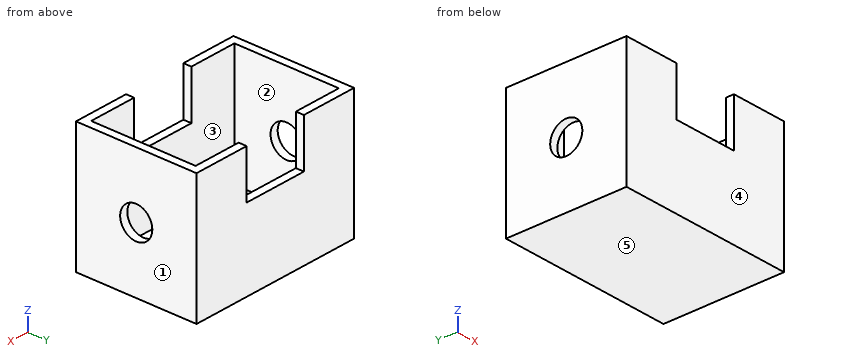
```python
from build123d import *

# Parameters (mm, degrees)
F0_W     = 139.7
F0_H     = 95.25
F1_DEPTH = 101.6
F2_T     = -6.35
F3_W     = 50.8
F3_H     = 38.1
F4_DEPTH = 101.6
F5_R     = 12.7
F6_DEPTH = 177.8


with BuildPart() as f1:
    # F0 (on Top) → F1 (new body)
    with BuildSketch(Plane.XY):
        Rectangle(F0_W, F0_H)
    extrude(amount=F1_DEPTH)

    # F2
    f2_openings = [f1.faces().sort_by_distance(p)[0] for p in [
        (0, 0, 101.6),
    ]]
    offset(amount=F2_T, openings=f2_openings)

    # F3 (on face) → F4 (cut)
    with BuildSketch(Plane.XZ.offset(47.625)):
        with Locations((0, 82.55)):
            Rectangle(F3_W, F3_H)
    extrude(amount=-F4_DEPTH, mode=Mode.SUBTRACT)

    # F5 (on face) → F6 (cut)
    with BuildSketch(Plane.YZ.offset(69.85)):
        with Locations((0, 50.8)):
            Circle(F5_R)
    extrude(amount=-F6_DEPTH, mode=Mode.SUBTRACT)


solid = f1.part
```
Geometry: final body of the model. Coordinates: model frame, mm. Face numbers are marked on the shaded views. A direction names the side the tool comes from. Coordinates: 2 decimals unless noted, no trailing zeros. Order: outer loops, then holes, each group sorted by start corner. A loop starts at its lowest first (then second) coordinate and runs counter-clockwise, first axis right, second up. Notation, with made-up numbers: (-0.5, 27.5) - (44.5, 27.5) arc R26 cw to (44.5, 41.5) - close; hole circle Ø11 at (73.5, 53). An arc over 180 degrees is marked (long way). Write each question's results on one line, items separated by ' | '.
(1) Line query: line 1 (X direction, y = 35.5, z = 52.5); line 2 (Z direction, x = -66.75, y = 0); line 3 (Y direction, x = -55, z = 81) (3 decimals). Output: solid intervals per line, ascending. Write a range as [from, to].
Values found:
line 1: x = [-69.85, -63.5], [63.5, 69.85] | line 2: z = [0, 38.1], [63.5, 101.6] | line 3: y = [-47.625, -41.275], [41.275, 47.625]
(2) First-contact query: pin 1 Ø3 at (x, y) = (-4.5, -44.5) entering from +Z; pin 2 Ø6 at (x, y) = (37, -7) entering from -Z. Flat tips, straight axial feed; report the tip coordinate or a pass-through.
Values found:
pin 1: stops at z = 63.5 | pin 2: stops at z = 0
(3) Section query B-B, the plane z = 50.8. Return the cut outline in (x, y) (3 decimals), plus the area to 3 significant figures.
Values found:
outline: (-69.85, -47.625) - (69.85, -47.625) - (69.85, -12.7) - (63.5, -12.7) - (63.5, -41.275) - (-63.5, -41.275) - (-63.5, -12.7) - (-69.85, -12.7) - close; (-69.85, 12.7) - (-63.5, 12.7) - (-63.5, 41.275) - (63.5, 41.275) - (63.5, 12.7) - (69.85, 12.7) - (69.85, 47.625) - (-69.85, 47.625) - close | area: 2,500 mm²
(4) Mould query, pull axis Y, two halves, no side actions, for the marked faces 3, 4 and 5. Classes: +Y half, -Y half, draft (parallel to the pull), parting line (faces both ways), or undercut.
Values found:
face 3: undercut | face 4: -Y half | face 5: draft
(5) Section query A-A, the plane y = 0. Return the cut outline in (x, z), plus the area to 3 significant figures.
Values found:
outline: (-69.85, 0) - (69.85, 0) - (69.85, 38.1) - (63.5, 38.1) - (63.5, 6.35) - (-63.5, 6.35) - (-63.5, 38.1) - (-69.85, 38.1) - close; (-69.85, 63.5) - (-63.5, 63.5) - (-63.5, 101.6) - (-69.85, 101.6) - close; (63.5, 63.5) - (69.85, 63.5) - (69.85, 101.6) - (63.5, 101.6) - close | area: 1,770 mm²
(6) Set-up query: the marked faces 1 and 2. Return all of +Z, -Z, +X, -X, +Y, -Y with unobstructed straight access to the full face (end or side cutting, diameter ignored); none if empty.
Values found:
face 1: +Z, -Z, +X, +Y, -Y | face 2: +Z
(7) Section query D-D, the plane x = -49. Return the cut outline in (y, z) (3 decimals), plus the area to 3 significant figures.
Values found:
outline: (-47.625, 0) - (47.625, 0) - (47.625, 101.6) - (41.275, 101.6) - (41.275, 6.35) - (-41.275, 6.35) - (-41.275, 101.6) - (-47.625, 101.6) - close | area: 1,810 mm²
(8) Section query C-C, the plane z = 28. Return the cut outline in (x, y) (3 decimals), plus the area to 3 significant figures.
Values found:
outline: (-69.85, -47.625) - (69.85, -47.625) - (69.85, 47.625) - (-69.85, 47.625) - close; hole (-63.5, -41.275) - (63.5, -41.275) - (63.5, 41.275) - (-63.5, 41.275) - close | area: 2,820 mm²
